Part model, mm, in its own coordinate system. A direction names the side the tool comes from. Round coordinates to 2 decimals unless told otherwise and drop trailing zeros. Write each loop counter-clockwise with the first axis right and the second up, starting at its lowest first coordinate (ties: lowest second). Pieces come first, ordered by that corner, then holes. Notation, with made-up numbers: (40, 38.5) -> (78, 38.5) arc R5 ccw to (78, 45.5) -> close; hole circle Ø9 at (58, -40). An arc over 180 degrees is marked (long way). Return JSON: item names as keys, results as strings. Group by question number.
(1) Tool access for faces 4 (the flat face through (-14.8, 0, 4)), 5 (the cylindrical face through (10.787, -0.102, 1.748)): list every direction of +Z, -Z, +X, -X, +Y, -Y with a clear straight run to the whole face (end or side of a thin tool).
(2) Drill centre lines: L1, parallel to Z at x = -2, y = -0.25; L2, parallel to X at y = -6.5, z = 1; L3, parallel to X at y = 3.5, z = 1.5. Where is each one in solid material? Low to high. Write a range as from..to.
(3) Saw through at B-B (x = -3.5). List the corners of the cut face in (y, z), plus the area to 3 significant figures.
(4) Mould opens along X. For faces 1 (the flat face through (14.8, 0, 4)), 2 (the flat face through (0, 0, 2.5)), 3 (the flat face through (0, 7.3, 5)) say: +X half, -X half, draft (parallel to the pull), parting line (faces both ways), or undercut.
(5) Saw through at A-A (y = 2.75). List the corners of the cut face in (x, z).
(6) Drop a flat-ended pin along its axis: pin 1 Ø7.5 at (x, y) = (4.5, -2.5) entering from -Z. Give the stop position or say it passes through.
Autodesk Inventor part; units mm, degrees
ref_plane "YZ Plane" through (0, 0, 0) normal (1, 0, 0) x (0, 1, 0)
ref_plane "XZ Plane" through (0, 0, 0) normal (0, 1, 0) x (-1, 0, 0)
ref_plane "XY Plane" through (0, 0, 0) normal (0, 0, 1) x (1, 0, 0)
sketch "Náčrt1" plane through (0, 0, 0) normal (0, 0, 1) x (1, 0, 0)
  line L0 (-20.72, 0) -> (20.72, 0)
  line L1 (0, -10.22) -> (0, 10.22)
  line L2 (-14.8, 7.3) -> (14.8, 7.3)
  line L3 (14.8, 7.3) -> (14.8, -7.3)
  line L4 (14.8, -7.3) -> (-14.8, -7.3)
  line L5 (-14.8, -7.3) -> (-14.8, 7.3)
  point P0 (0, 0)
  point P1 (0, 7.3)
  point P2 (14.8, 0)
  dimension "d0" = 29.6
  dimension "d1" = 14.6
extrude "Vysunutí1" add sketch "Náčrt1" along normal blind 7.8
sketch "Náčrt2" plane through (-14.8, -7.3, 0) normal (0, -1, 0) x (1, 0, 0)
  line L0 (0, 0) -> (29.6, 0)
  line L1 (29.6, 0) -> (29.6, 7.8)
  line L2 (0, 7.8) -> (29.6, 7.8)
  line L3 (0, 0) -> (0, 7.8)
  point P0 (14.8, 0)
  point P1 (14.8, 0)
hole "Díra1" at (0, -7.3, 0) direction (0, 1, 0) diameter 5 end through all
sketch "Náčrt3" plane through (-14.8, -7.3, 7.8) normal (0, -1, 0) x (1, 0, 0)
  line L0 (5.8, -7.8) -> (23.8, -7.8) construction
  line L1 (17.3, -7.8) -> (29.6, -7.8)
  line L2 (5.8, -10.3) -> (23.8, -10.3)
  line L3 (23.8, -5.3) -> (5.8, -5.3)
  arc A0 (5.8, -5.3) -> (5.8, -10.3) centre (5.8, -7.8) ccw
  arc A1 (23.8, -10.3) -> (23.8, -5.3) centre (23.8, -7.8) ccw
  point P0 (14.8, -7.8)
  dimension "d14" = 9
  dimension "d15" = 2.5
extrude "Vysunutí2" cut sketch "Náčrt3" against normal through all
properties part number "drzak_kable_guma"
Computed values:
{
 "1": {"face 4": "+Z, -Z, -X, +Y, -Y", "face 5": "-Z, +Y, -Y"},
 "2": {"L1": "2.5..7.8", "L2": "-14.8..-11.29, 11.29..14.8", "L3": "-14.8..-11, 11..14.8"},
 "3": {"outline": "(-7.3, 2.5) -> (7.3, 2.5) -> (7.3, 7.8) -> (-7.3, 7.8) -> close", "area": "77.4 mm2"},
 "4": {"face 1": "+X half", "face 2": "undercut", "face 3": "draft"},
 "5": {"outline": "(-14.8, 0) -> (-11.5, 0) arc R2.5 cw to (-9, 2.5) -> (9, 2.5) arc R2.5 cw to (11.5, 0) -> (14.8, 0) -> (14.8, 7.8) -> (-14.8, 7.8) -> close"},
 "6": {"pin 1": "z = 2.5"}
}
